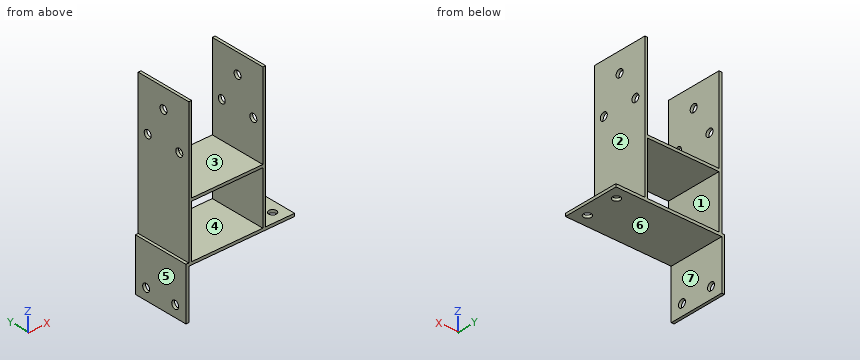
```python
from build123d import *

# Parameters (mm, degrees)
F1_W     = 101
F1_H     = 4
F2_DEPTH = 80
F3_R     = 5.5
F5_DEPTH = 25
F4_R     = 5.5
F6_DEPTH = 25
F7_R     = 5.5
F8_DEPTH = 113.001


with BuildPart() as f2:
    # F0 (on Front) + F1 (on face) → F2 (new body)
    with BuildSketch(Plane.XZ):
        Polygon((0, -70), (0, 0), (150, 0), (150, 4), (-4, 4), (-4, -70), align=None)
    with BuildSketch(Plane.XZ):
        Polygon((0, 4), (4, 4), (4, 79), (4, 83), (4, 204), (0, 204), align=None)
        with Locations((54.5, 81)):
            Rectangle(F1_W, F1_H)
        Polygon((105, 79), (105, 4), (109, 4), (109, 204), (105, 204), (105, 83), align=None)
    extrude(amount=F2_DEPTH)

    # F3 (on face) → F5 (cut)
    with BuildSketch(Plane.XY.offset(4)):
        with Locations((134, -17)):
            Circle(F3_R)
        with Locations((134, -63)):
            Circle(F3_R)
    extrude(amount=-F5_DEPTH, mode=Mode.SUBTRACT)

    # F4 (on face) → F6 (cut)
    with BuildSketch(Plane(origin=(-4, 0, 0), x_dir=(0, -1, 0), z_dir=(-1, 0, 0))):
        with Locations((17, -54)):
            Circle(F4_R)
        with Locations((63, -54)):
            Circle(F4_R)
    extrude(amount=-F6_DEPTH, mode=Mode.SUBTRACT)

    # F7 (on face) → F8 (cut, through all)
    with BuildSketch(Plane.YZ.offset(109)):
        with Locations((-40, 176)):
            Circle(F7_R)
        with Locations((-15, 134)):
            Circle(F7_R)
        with Locations((-65, 134)):
            Circle(F7_R)
    extrude(amount=-F8_DEPTH, mode=Mode.SUBTRACT)


solid = f2.part
```
Verification items for the finished model (mm, model axes). Face numbers are marked on the shaded views. A direction names the side the tool comes from. Give positions to 0.01 mm unless a question says otherwise; leave off trailing zeros. Loops run counter-clockwise (first coordinate to the right, second up) from the corner with the lowest first, then second, coordinate; pieces in that order, holes last. Notation, with made-up numbers: M -37,42.5 L -26,42.5 A4 ccw -26,46.5 Z; hole C 22,83.25 d9. An arc over 180 degrees is marked long. One line per question, with ' | ' between items.
Item 1: Section check B-B, the plane x = 93. Record the cut outline in (y, z).
Completed:
outline: M -80,0 L 0,0 L 0,4 L -80,4 Z; M -80,79 L 0,79 L 0,83 L -80,83 Z
Item 2: Depth check by flat-ended pin: P1, Ø2, axis at y = -36.5, z = 96.5, coming from the +X side; P2, Ø17.5, axis at x = 134, y = -17, coming from the -Z side; P3, Ø3, axis at x = 82, y = -66.5, coming from the +Z side; P4, Ø4.5, axis at x = -2, y = -38.5, coming from the +Z side. Enter the tip coordinate at first touch or a pass-through.
Completed:
P1: stops at x = 109 | P2: stops at z = 0 | P3: stops at z = 83 | P4: stops at z = 204
Item 3: Section check A-A, the plane z = 176. Record the cut outline in (x, y), plus the area to 3 significant figures.
Completed:
outline: M 0,-80 L 4,-80 L 4,-45.5 L 0,-45.5 Z; M 0,-34.5 L 4,-34.5 L 4,0 L 0,0 Z; M 105,-80 L 109,-80 L 109,-45.5 L 105,-45.5 Z; M 105,-34.5 L 109,-34.5 L 109,0 L 105,0 Z | area: 552 mm^2
Item 4: Section check D-D, the plane z = 107.5. Record the cut outline in (x, y).
Completed:
outline: M 0,-80 L 4,-80 L 4,0 L 0,0 Z; M 105,-80 L 109,-80 L 109,0 L 105,0 Z
Item 5: Tool access check on the marked faces 1, 2 and 3. Record the directions out of +Z, -Z, +X, -X, +Y, -Y that give a thin tool (end or side, any length) a straight path to the whole face; none if there is none.
Completed:
face 1: +Y, -Y | face 2: +Z, +X, +Y, -Y | face 3: +Z, +Y, -Y
Item 6: Thickness scan on line 1 (Y direction, x = 134, z = 1.95); line 2 (Z direction, x = 104.5, y = -21.5); line 3 (X direction, y = -63, z = 141). Record the ranges inside material, lowest first. Write a range as [from, to].
Completed:
line 1: y = [-80, -68.5], [-57.5, -22.5], [-11.5, 0] | line 2: z = [0, 4], [79, 83] | line 3: x = [0, 4], [105, 109]
Item 7: Draft check along X on the marked faces 4, 5, 6 and 7. Enter one of: +X half, -X half, draft (parallel to the pull), parting line (faces both ways), or undercut.
Completed:
face 4: undercut | face 5: -X half | face 6: draft | face 7: +X half
Item 8: Section check C-C, the plane y = -17. State how many separate pieces and enclosed holes the cut face has, plus the area to 3 significant figures.
Completed:
separate pieces: 5 | enclosed holes: 1 | area: 2,730 mm^2
